Could you check a few things on this drawing? It's one solid part, dimensions in mm from its lowest x, y, z. A direction names the side the tool comes from. Round coordinates to 2 decimals unless told otherwise and drop trailing zeros. Write each loop counter-clockwise with the first axis right and the second up, starting at its lowest first coordinate (ties: lowest second). Pieces come first, ordered by that corner, then holes. Notation, with made-up numbers: M -13,-6 L 22,-6 A11 ccw 22,0 Z; hole C 0.5,13.25 d11. An arc over 180 degrees is marked long. One line per item, written item: value. Start each with the question number.
(1) I want a section at D-D on y = 116. Please give me the cut outline in (x, z), and give its area (3 significant figures).
(2) I want a section at A-A on z = 123. Please give me the cut outline in (x, y).
(3) I want a section at C-C on y = 70. Please give me the cut outline in (x, z), and give its area (3 significant figures).
(4) If I drill on L1, parallel to Y at x = 64, z = 114; L2, parallel to Z at x = 67, y = 76; L3, parallel to X at y = 130.5, z = 136, over which ranges is the centre line in solid material (lowest first)?
(5) I want a section at B-B on x = 60.5. Please give me the cut outline in (y, z), and give its area (3 significant figures).
(6) Which directions (+Z, -Z, +X, -X, +Y, -Y) give clear straight access to the entire face, cutting with the end or side of a thin tool? Please do the marked faces 1 and 2.
(7) I'm going to push flat-ended pins straight in: pin 1 Ø12 at (y, z) = (31.5, 31.5) entering from -X; pin 2 Ø1 at (x, y) = (8.5, 83) entering from -Z; pin 3 Ø5 at (x, y) = (10, 85) entering from +Z. Where does each tip first touch, or does it pass through?
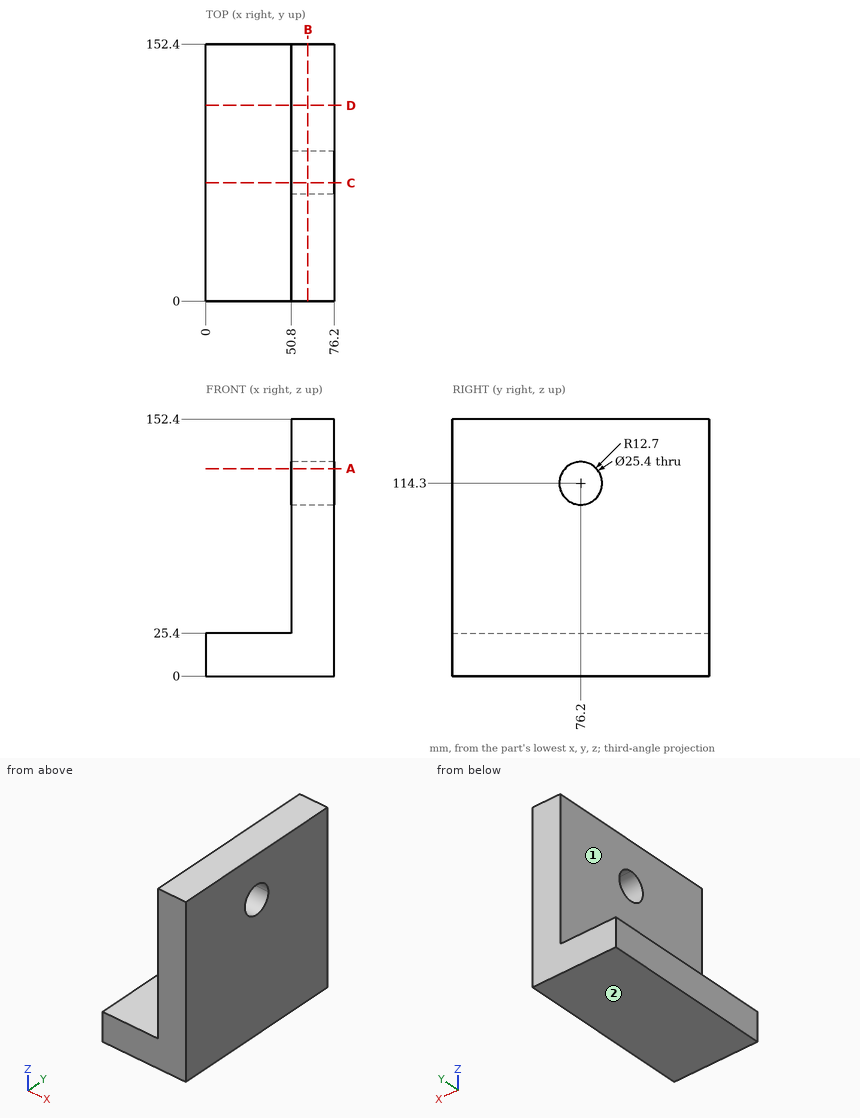
Found:
1. outline: M 0,0 L 76.2,0 L 76.2,152.4 L 50.8,152.4 L 50.8,25.4 L 0,25.4 Z
1. area: 5,160 mm²
2. outline: M 50.8,0 L 76.2,0 L 76.2,66.95 L 50.8,66.95 Z; M 50.8,85.45 L 76.2,85.45 L 76.2,152.4 L 50.8,152.4 Z
3. outline: M 0,0 L 76.2,0 L 76.2,103.22 L 50.8,103.22 L 50.8,25.4 L 0,25.4 Z; M 50.8,125.38 L 76.2,125.38 L 76.2,152.4 L 50.8,152.4 Z
3. area: 4,600 mm²
4. L1: y = 0 to 63.5, 88.9 to 152.4
4. L2: z = 0 to 101.6, 127 to 152.4
4. L3: x = 50.8 to 76.2
5. outline: M 0,0 L 152.4,0 L 152.4,152.4 L 0,152.4 Z; hole C 76.2,114.3 d25.4
5. area: 22,700 mm²
6. face 1: +Z, -X, +Y, -Y
6. face 2: -Z, +X, -X, +Y, -Y
7. pin 1: stops at x = 50.8
7. pin 2: stops at z = 0
7. pin 3: stops at z = 25.4
